```python
from build123d import *

# Parameters (mm, degrees)
SKETCH2_W           = 180
SKETCH2_H           = 20
BOSS_EXTRUDE1_DEPTH = 30
SKETCH3_R           = 12.5
CUT_EXTRUDE2_DEPTH  = 31
SKETCH5_R           = 12.5
BOSS_EXTRUDE4_DEPTH = 5


with BuildPart() as part:
    # Sketch2 → Boss-Extrude1 (new body)
    with BuildSketch(Plane(origin=(0, 0, 0), x_dir=(0, 0, -1), z_dir=(1, 0, 0))):
        with Locations((90, 10)):
            Rectangle(SKETCH2_W, SKETCH2_H)
    extrude(amount=-BOSS_EXTRUDE1_DEPTH)

    # Sketch3 → Cut-Extrude2 (cut, through all)
    with BuildSketch(Plane(origin=(0, 0, 0), x_dir=(0, 0, -1), z_dir=(1, 0, 0))):
        with Locations((170, 27.5)):
            Circle(SKETCH3_R)
    extrude(amount=-CUT_EXTRUDE2_DEPTH, mode=Mode.SUBTRACT)

    # Sketch5 → Boss-Extrude4 (add, symmetric)
    with BuildSketch(Plane(origin=(-15, 0, 0), x_dir=(0, 0, -1), z_dir=(1, 0, 0))):
        with Locations((170, 27.5)):
            Circle(SKETCH5_R)
    extrude(amount=BOSS_EXTRUDE4_DEPTH, both=True)


solid = part.part
```
Input: part model. Units: mm. Frame: model coordinates. A direction names the side the tool comes from. Give positions to 0.01 mm unless a question says otherwise; leave off trailing zeros. Write each loop counter-clockwise with the first axis right and the second up, starting at its lowest first coordinate (ties: lowest second). Pieces come first, ordered by that corner, then holes. Notation, with made-up numbers: (71.25, 70.25) - (97.25, 70.25) arc R34 ccw to (97.25, 100.25) - close; hole circle Ø2 at (77.25, 43.25). An arc over 180 degrees is marked (long way). Write item = value, one per line. Start each with the question number.
1. Mould query, pull axis Z, two halves, no side actions, for faces 1 (the flat face through (0, 10, -89)), 2 (the flat face through (-20, 28, -170)), 3 (the flat face through (-15, 10, 0)), 4 (the cylindrical face through (-25, 15, -170)). Classes: released by +Z, released by -Z, zero draft, split by the parting line, or undercut.
2. Section query A-A, the plane x = -27. Output: boundary loops of the cut face in (y, z), then the cut area to 3 significant figures.
3. Section query C-C, the plane y = 24. Output: boundary loops of the cut face in (x, z), then the cut area to 3 significant figures.
4. Ray query, L1, parallel to Z at x = -15.5, y = 12; L2, parallel to Y at x = -6, z = -49.5; L3, parallel to Y at x = -10.5, z = -170.5. Return the intervals inside material, ascending.
5. Section query B-B, the plane z = -170. Output: boundary loops of the cut face in (x, y).
6. First-contact query: pin 1 Ø6 at (x, y) = (-15.5, 13.5) entering from -Z; pin 2 Ø1.5 at (x, z) = (-4, -58.5) entering from +Y. Flat tips, straight axial feed; report the tip coordinate or a pass-through.
7. Section query D-D, the plane z = -149. Output: boundary loops of the cut face in (x, y).
8. Access query for faces 5 (the flat face through (-15, 10, -180)), 6 (the flat face through (-30, 10, -89)), 7 (the flat face through (-10, 28, -170)). Directions: +Z, -Z, +X, -X, +Y, -Y. A direction counts if a zero-diameter tool reaches every point of the face in a straight line with its end or side. Return the directions, or none.
Check sheet entries:
q1.face_1 = zero draft
q1.face_2 = undercut
q1.face_3 = released by +Z
q1.face_4 = undercut
q2.outline = (0, -180) - (20, -180) arc R12.5 cw to (20, -160) - (20, 0) - (0, 0) - close
q2.area = 3,530 mm2
q3.outline = (-20, -182) - (-10, -182) - (-10, -158) - (-20, -158) - close
q3.area = 240 mm2
q4.L1 = -180 to 0
q4.L2 = 0 to 20
q4.L3 = 0 to 39.99
q5.outline = (-30, 0) - (0, 0) - (0, 15) - (-10, 15) - (-10, 40) - (-20, 40) - (-20, 15) - (-30, 15) - close
q6.pin_1 = -180
q6.pin_2 = 20
q7.outline = (-30, 0) - (0, 0) - (0, 20) - (-30, 20) - close
q8.face_5 = -Z, +X, -X, -Y
q8.face_6 = +Z, -Z, -X, +Y, -Y
q8.face_7 = +X, +Y
